Can you work these out from the drawing? Everything is in mm from the part's minimum corner. A direction names the side the tool comes from. Coordinates: 2 decimals unless noted, no trailing zeros. Loops run counter-clockwise (first coordinate to the right, second up) from the corner with the lowest first, then second, coordinate; pieces in that order, holes last. Notation, with made-up numbers: (-24.5, 17) - (34.5, 17) arc R24 cw to (34.5, 42) - close; hole circle Ø4 at (70, 66). An arc over 180 degrees is marked (long way). Put each result on its own line as item: value. Start each with the question number.
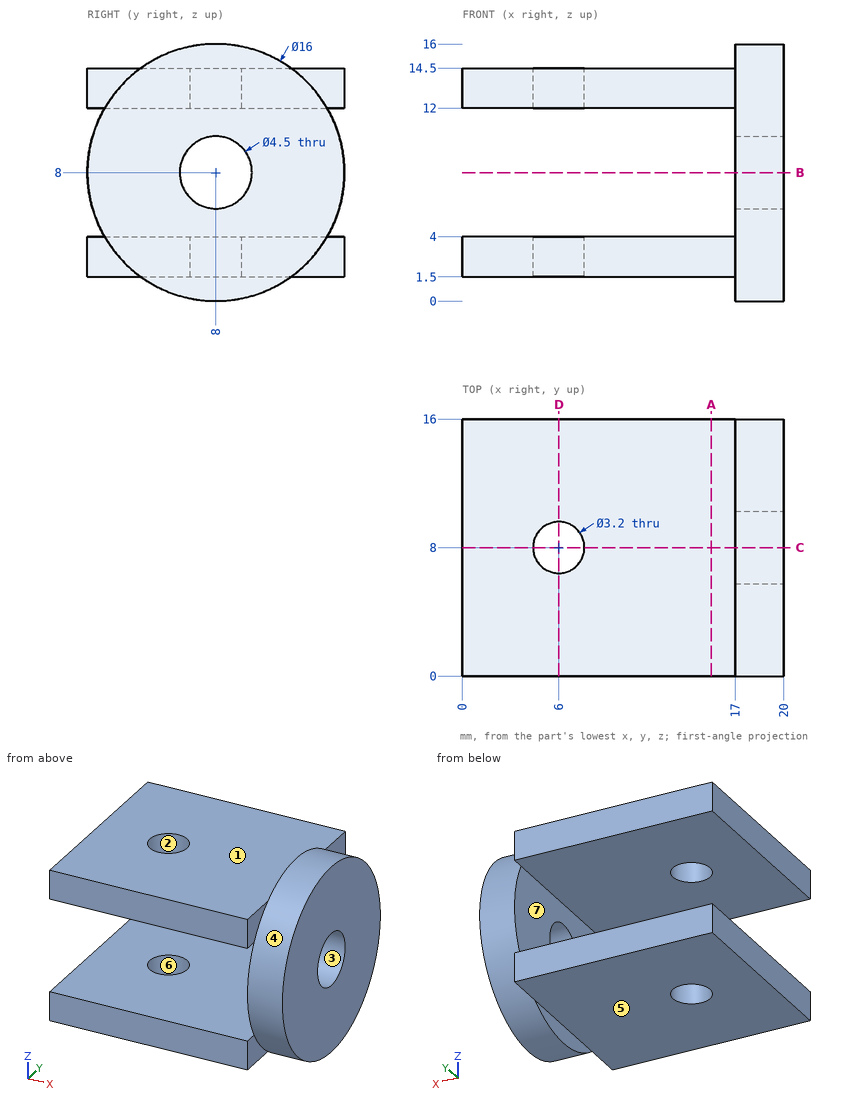
Q1. I want a section at A-A on x = 15.5. List the corners of the cut face in (y, z) for me, and give its area (3 significant figures).
Q2. We'd pull the mould along Z, two halves only. Please class the marked faces 1, 2, 3 and 4: released by +Z, released by -Z, zero draft, split by the parting line, or undercut.
Q3. I want a section at C-C on y = 8. List the corners of the cut face in (x, z) for me, and give its area (4 significant figures).
Q4. Will these pins go through, and if not, where does the flat tip stop? pin 1 (1 mm diameter, centred on x = 18, y = 13.5, fed in from -Z) (3 decimals); pin 2 (5 mm diameter, centred on x = 11.5, y = 5.5, fed in from -Z); pin 3 (1.2 mm diameter, centred on y = 10, z = 15.5, fed in from -X).
Q5. I want a section at D-D on x = 6. List the corners of the cut face in (y, z) for me, and give its area (3 significant figures).
Q6. I want a section at B-B on z = 8. List the corners of the cut face in (x, y) for me, and give its area (3 significant figures).
Q7. On a 3-axis mill with a long thin cutter (end or side, diameter ignored), from which of +Z, -Z, +X, -X, +Y, -Y can I reach the whole of each face in a straight line? I mean the marked faces 5, 6 and 7. Say none if no direction works.
Q8. Please list where these lines run through material, in increasing order: line 1 along Z through (x, y) = (17.75, 8); line 2 along Z through (x, y) = (6, 11.5); line 3 along Y through (x, z) = (6, 13.15). Write a range as [from, to].
Calculated:
1. outline: (0, 1.5) - (16, 1.5) - (16, 4) - (0, 4) - close; (0, 12) - (16, 12) - (16, 14.5) - (0, 14.5) - close
1. area: 80.0 mm2
2. face 1: released by +Z
2. face 2: zero draft
2. face 3: undercut
2. face 4: split by the parting line
3. outline: (0, 1.5) - (4.4, 1.5) - (4.4, 4) - (0, 4) - close; (0, 12) - (4.4, 12) - (4.4, 14.5) - (0, 14.5) - close; (7.6, 1.5) - (17, 1.5) - (17, 0) - (20, 0) - (20, 5.75) - (17, 5.75) - (17, 4) - (7.6, 4) - close; (7.6, 12) - (17, 12) - (17, 10.25) - (20, 10.25) - (20, 16) - (17, 16) - (17, 14.5) - (7.6, 14.5) - close
3. area: 103.5 mm2
4. pin 1: z = 1.755
4. pin 2: z = 1.5
4. pin 3: x = 17
5. outline: (0, 1.5) - (6.4, 1.5) - (6.4, 4) - (0, 4) - close; (0, 12) - (6.4, 12) - (6.4, 14.5) - (0, 14.5) - close; (9.6, 1.5) - (16, 1.5) - (16, 4) - (9.6, 4) - close; (9.6, 12) - (16, 12) - (16, 14.5) - (9.6, 14.5) - close
5. area: 64.0 mm2
6. outline: (17, 0) - (20, 0) - (20, 5.75) - (17, 5.75) - close; (17, 10.25) - (20, 10.25) - (20, 16) - (17, 16) - close
6. area: 34.5 mm2
7. face 5: -Z, -X, +Y, -Y
7. face 6: +Z, -Z
7. face 7: -X, +Y, -Y
8. line 1: [0, 5.75], [10.25, 16]
8. line 2: [1.5, 4], [12, 14.5]
8. line 3: [0, 6.4], [9.6, 16]
